```python
from build123d import *

# Parameters (mm, degrees)
F1_DEPTH = 38.1
F2_R     = 6.35
F3_DEPTH = 50.801
F4_R     = 3.175
F5_DEPTH = 50.8


with BuildPart() as f1:
    # F0 (on Top) → F1 (new body)
    with BuildSketch(Plane.XY):
        Polygon((0, 50.8), (0, 0), (12.7, 0), (12.7, 50.8), (6.35, 50.8), align=None)
        with BuildLine():
            Line((12.7, 0), (0, 0))
            ThreePointArc((0, 0), (-12.7, -12.7), (-25.4, 0))
            ThreePointArc((-25.4, 0), (-31.75, 6.35), (-38.1, 0))
            ThreePointArc((-38.1, 0), (-12.7, -25.4), (12.7, 0))
        make_face()
        Polygon((-19.05, 50.8), (0, 50.8), (6.35, 50.8), (6.35, 63.5), (-19.05, 63.5), align=None)
        Polygon((6.35, 50.8), (12.7, 50.8), (31.75, 50.8), (31.75, 63.5), (6.35, 63.5), align=None)
    extrude(amount=F1_DEPTH)

    # F2 (on face) → F3 (cut, through all)
    with BuildSketch(Plane.YZ.offset(12.7)):
        with Locations((25.4, 19.05)):
            Circle(F2_R)
    extrude(amount=-F3_DEPTH, mode=Mode.SUBTRACT)

    # F4 (on face) → F5 (cut)
    with BuildSketch(Plane(origin=(0, 63.5, 0), x_dir=(-1, 0, 0), z_dir=(0, 1, 0))):
        with Locations((-6.35, 19.05)):
            Circle(F4_R)
    extrude(amount=-F5_DEPTH, mode=Mode.SUBTRACT)


solid = f1.part
```
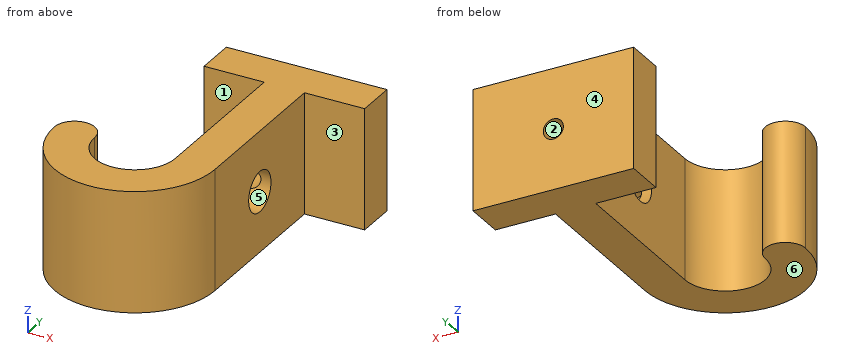
Here's how the part is built. I have some questions about the finished solid (model axes, mm). Face numbers are marked on the shaded views. A direction names the side the tool comes from. Give positions to 0.01 mm unless a question says otherwise; leave off trailing zeros. Order: outer loops, then holes, each group sorted by start corner. A loop starts at its lowest first (then second) coordinate and runs counter-clockwise, first axis right, second up. Notation, with made-up numbers: M 1,36.5 L 25,36.5 A28 ccw 25,64.5 Z; hole C -32,-11 d3. An arc over 180 degrees is marked long. Use a Markdown table: item, result. Add a question column.
1. Suppose I cut it at D-D (y = 39). List the corners of the cut face in (x, z) for me (3 decimals), and give its area (3 significant figures).
2. On a 3-axis mill with a long thin cutter (end or side, diameter ignored), from which of +Z, -Z, +X, -X, +Y, -Y can I reach the whole of each face in a straight line? I mean the marked faces 1, 2 and 3. Say none if no direction works.
3. If we mould it in two halves opening along Z, with no side actions, what happens to the marked faces 4, 5 and 6? For each: +Z half, -Z half, draft (parallel to the pull), parting line (faces both ways), or undercut.
4. Suppose I cut it at B-B (z = 19.05). List the corners of the cut face in (x, y) for me (3 decimals).
5. Suppose I cut it at A-A (y = 25.4). List the corners of the cut face in (x, z) for me, and give its area (3 significant figures).
6. Suppose I cut it at C-C (x = -12.7). List the corners of the cut face in (y, z) for me, and give its area (3 significant figures).
7. For pin 1 Ø1 at (x, y) = (14.5, 6) entering from +Z; pin 2 Ø10 at (x, z) = (6.35, 19.05) entering from -Y; pin 3 Ø4 at (x, z) = (-20.5, 15.5) entering from -Y; pin 4 Ø15 at (x, z) = (-9.5, 24.5) entering from -Y, each with a flat end and sliding along its axis, tell me the tip position at first contact or that it passes through.
8. I need wall thicknesses on probe 1 along X at (y, z) = (56, 19); probe 2 along X at (y, z) = (33, 19); probe 3 along Z at (x, y) = (6.35, 14.75) (3 decimals). Which ranges of each line are inside material? Lowest first, please. Write a range as from..to.
Results list:
| question | item | result |
|---|---|---|
| 1 | outline | M 0,0 L 12.7,0 L 12.7,38.1 L 0,38.1 Z; hole C 6.35,19.05 d6.35 |
| 1 | area | 452 mm² |
| 2 | face 1 | +Z, -Z, -X |
| 2 | face 2 | +Y |
| 2 | face 3 | +Z, -Z, +X, -Y |
| 3 | face 4 | draft |
| 3 | face 5 | undercut |
| 3 | face 6 | -Z half |
| 4 | outline | M -38.1,0 A25.4 ccw 12.7,0 L 12.7,19.05 L 9.525,19.05 L 9.525,12.7 L 3.175,12.7 L 3.175,19.05 L 0,19.05 L 0,0 A12.7 cw -25.4,0 A6.35 ccw Z; M -19.05,50.8 L 0,50.8 L 0,31.75 L 3.175,31.75 L 3.175,63.5 L -19.05,63.5 Z; M 9.525,31.75 L 12.7,31.75 L 12.7,50.8 L 31.75,50.8 L 31.75,63.5 L 9.525,63.5 Z |
| 5 | outline | M 0,0 L 12.7,0 L 12.7,12.7 L 0,12.7 Z; M 0,25.4 L 12.7,25.4 L 12.7,38.1 L 0,38.1 Z |
| 5 | area | 323 mm² |
| 6 | outline | M -25.4,0 L -12.7,0 L -12.7,38.1 L -25.4,38.1 Z; M 50.8,0 L 63.5,0 L 63.5,38.1 L 50.8,38.1 Z |
| 6 | area | 968 mm² |
| 7 | pin 1 | passes through |
| 7 | pin 2 | stops at y = -21.16 |
| 7 | pin 3 | stops at y = -24.73 |
| 7 | pin 4 | stops at y = -25.4 |
| 8 | probe 1 | x = -19.05..3.18, 9.52..31.75 |
| 8 | probe 2 | x = 0..3.18, 9.52..12.7 |
| 8 | probe 3 | z = 0..15.875, 22.225..38.1 |
